```python
from build123d import *

# Parameters (mm, degrees)
SKETCH1_R             = 0.5
SKETCH1_R_2           = 3.4
SKETCH1_R_3           = 2.2
SKETCH1_R_4           = 1.25
BASE_DEPTH            = 2.08
SKETCH1_3_R           = 3.4
SKETCH1_3_R_2         = 2.2
CONNECTION_DEPTH      = 2.5
CONNECTION_DEPTH_BACK = 2.25


with BuildPart() as part:
    # Sketch1 → Base (new body)
    with BuildSketch(Plane.XY):
        with BuildLine():
            ThreePointArc((16.424, -1.942221409), (18.2, 0), (16.424, 1.942221409))
            Line((16.424, 1.942221409), (0.303384615, 3.386437328))
            ThreePointArc((0.303384615, 3.386437328), (2.509134083, 2.294394507), (3.4, 0))
            ThreePointArc((3.4, 0), (2.509134083, -2.294394507), (0.303384615, -3.386437328))
            Line((0.303384615, -3.386437328), (16.424, -1.942221409))
        make_face()
        with Locations((5.1, 0)):
            Circle(SKETCH1_R, mode=Mode.SUBTRACT)
        with Locations((6.983333333, 0)):
            Circle(SKETCH1_R, mode=Mode.SUBTRACT)
        with Locations((8.866666667, 0)):
            Circle(SKETCH1_R, mode=Mode.SUBTRACT)
        with Locations((10.75, 0)):
            Circle(SKETCH1_R, mode=Mode.SUBTRACT)
        with Locations((12.633333333, 0)):
            Circle(SKETCH1_R, mode=Mode.SUBTRACT)
        with Locations((14.516666667, 0)):
            Circle(SKETCH1_R, mode=Mode.SUBTRACT)
        with Locations((16.4, 0)):
            Circle(SKETCH1_R, mode=Mode.SUBTRACT)
        Circle(SKETCH1_R_2)
        Circle(SKETCH1_R_3, mode=Mode.SUBTRACT)
        Circle(SKETCH1_R_3)
        Circle(SKETCH1_R_4, mode=Mode.SUBTRACT)
    extrude(amount=BASE_DEPTH)

    # Sketch1_3 → Connection (add, two sides)
    with BuildSketch(Plane.XY) as connection_sk:
        Circle(SKETCH1_3_R)
        Circle(SKETCH1_3_R_2, mode=Mode.SUBTRACT)
    extrude(amount=CONNECTION_DEPTH)
    extrude(connection_sk.sketch, amount=-CONNECTION_DEPTH_BACK)


solid = part.part
```
The listing builds one solid part. Answer for the finished solid, in the listing's coordinates (mm). A direction names the side the tool comes from. Give positions to 0.01 mm unless a question says otherwise; leave off trailing zeros. Order: outer loops, then holes, each group sorted by start corner. A loop starts at its lowest first (then second) coordinate and runs counter-clockwise, first axis right, second up.
1) Consider line 1 along Y through (x, z) = (16.4, 1.65); line 2 along Y through (x, z) = (0, 1.5); line 3 along Z through (x, y) = (14.25, -1). Determine where each line is inside the solid, lowest interval first.
Reported:
line 1: y = -1.94 to -0.5, 0.5 to 1.94
line 2: y = -3.4 to -1.25, 1.25 to 3.4
line 3: z = 0 to 2.08
2) Determine the mould class of faces 1 (the face through (6.484, 0.022, 1.025)), 2 (the face through (-2, 2, 2.5)), 3 (the face through (-3.4, 0.1, 0.2)) for opening direction Y: pulls with the +Y half, pulls with the -Y half, needs draft (parallel to the pull), parting line crosses it, or undercut.
Reported:
face 1: undercut
face 2: needs draft
face 3: parting line crosses it
3) Given P1, Ø4, axis at x = 11.5, y = -1.5, coming from the +Z side; P2, Ø1, axis at y = -2.5, z = 0.5, coming from the -X side; P3, Ø1.5, axis at x = 0, y = 0, coming from the +Z side, each flat-ended and moving along its own axis, determine where each tip first touches the part or whether it passes through.
Reported:
P1: stops at z = 2.08
P2: stops at x = -2.75
P3: passes through
4) Find section D-D on z = -0.75. Write down the section's boundary in (x, y).
Reported:
outline: circle Ø6.8 at (0, 0); hole circle Ø4.4 at (0, 0)
5) Find section B-B on z = 0.35. Give the number of separate pieces and of enclosed holes in the cut face, then the cut area to 3 significant figures.
Reported:
separate pieces: 1
enclosed holes: 8
area: 101 mm2
6) Find section C-C on y = 1. Write down the section's boundary in (x, z).
Reported:
outline: (-3.25, -2.25) - (-1.96, -2.25) - (-1.96, 0) - (-0.75, 0) - (-0.75, 2.08) - (-1.96, 2.08) - (-1.96, 2.5) - (-3.25, 2.5) - close; (0.75, 0) - (1.96, 0) - (1.96, -2.25) - (3.25, -2.25) - (3.25, 0) - (17.92, 0) - (17.92, 2.08) - (3.25, 2.08) - (3.25, 2.5) - (1.96, 2.5) - (1.96, 2.08) - (0.75, 2.08) - close
7) Find section A-A on x = 0. Write down the section's boundary in (y, z), then the cut area to 3 significant figures.
Reported:
outline: (-3.4, -2.25) - (-2.2, -2.25) - (-2.2, 0) - (-1.25, 0) - (-1.25, 2.08) - (-2.2, 2.08) - (-2.2, 2.5) - (-3.4, 2.5) - close; (1.25, 0) - (2.2, 0) - (2.2, -2.25) - (3.4, -2.25) - (3.4, 2.5) - (2.2, 2.5) - (2.2, 2.08) - (1.25, 2.08) - close
area: 15.4 mm2
8) For faces 4 (the face through (18.2, 0, 1)), 5 (the face through (2.1, 0.66, 2.29)), 6 (the face through (1, -1, 0)), determine the directions among +Z, -Z, +X, -X, +Y, -Y from which every point of the face is accessible in a straight line to the end or side of a thin tool.
Reported:
face 4: +Z, -Z, +X
face 5: +Z
face 6: -Z
